Solid Edge part; units mm, degrees
sketch "Sketch1" plane through (0, 0, 0) normal (0, -1, 0) x (1, 0, 0)
  line L0 (20, 36) -> (-16, 36)
  line L1 (-16, 36) -> (-16, -36)
  line L2 (-16, -36) -> (20, -36)
  line L3 (20, -36) -> (20, -40)
  line L4 (20, -40) -> (-20, -40)
  line L5 (-20, -40) -> (-20, 40)
  line L6 (-20, 40) -> (20, 40)
  line L7 (20, 40) -> (20, 36)
  dimension "D1" = 20
  dimension "D2" = 20
  dimension "D3" = 20
extrude "Protrusion1" add sketch "Sketch1" against normal blind 350
sketch "Sketch2" plane through (0, 175, 40) normal (0, 0, 1) x (0, 1, 0)
  line L0 (-175, 20) -> (-135, -20)
extrude "Cutout1" cut sketch "Sketch2" against normal through all material side at (0.0354, 19.9646, 40)
sketch "Sketch3" plane through (0, 175, 40) normal (0, 0, 1) x (0, 1, 0)
  line L0 (175, 20) -> (135, -20)
extrude "Cutout2" cut sketch "Sketch3" against normal through all material side at (0.0354, 330.0354, 40)
hole "Bohrung_1" at (-16, 142.5, 17) direction (-1, 0, 0) diameter 6 end up to next
hole "Hole1" at (-16, 207.5, 17) direction (-1, 0, 0) diameter 6 end up to next
hole "Bohrung_3" at (-16, 50, 15.6) direction (-1, 0, 0) diameter 5 end up to next
hole "Hole2" at (-16, 105, 15.6) direction (-1, 0, 0) diameter 5 end up to next
hole "Hole3" at (-16, 245, 15.6) direction (-1, 0, 0) diameter 5 end up to next
hole "Hole4" at (-16, 300, 15.6) direction (-1, 0, 0) diameter 5 end up to next
sketch "Sketch4" plane through (20, 175, -38) normal (1, 0, 0) x (0, 1, 0)
  line L0 (-25, -2) -> (25, -2)
  line L1 (25, -2) -> (25, 28)
  line L2 (25, 28) -> (-25, 28)
  line L3 (-25, 28) -> (-25, -2)
  dimension "D1" = 25
  dimension "D2" = 25
extrude "Cutout3" cut sketch "Sketch4" against normal through all
properties material "AlMgSi 0,5-1"
Geometry: final body of the model. Coordinates: model frame, mm. A direction names the side the tool comes from. Coordinates: 2 decimals unless noted, no trailing zeros. Order: outer loops, then holes, each group sorted by start corner. A loop starts at its lowest first (then second) coordinate and runs counter-clockwise, first axis right, second up.
(1) Material intervals for probe 1 along Z at (x, y) = (-18.6, 245); probe 2 along Z at (x, y) = (-16.9, 207.5); probe 3 along X at (y, z) = (230, 33), sorted ascending.
(2) Section query A-A (z = -23). Return the cut outline in (x, y).
(3) Section query C-C (x = -8). Return the cut outline in (y, z), plus the area to 3 significant figures.
(4) First-contact query: pin 1 (6 mm diameter, centred on y = 105, z = 15.6, fed in from +X); pin 2 (9 mm diameter, centred on x = -2, z = -32.5, fed in from +Y); pin 3 (2 mm diameter, centred on x = -17.5, y = 163.5, fed in from -Z). Flat tips, straight axial feed; report the tip coordinate or a pass-through.
(5) Draft query along Y for faces 4 (the face through (-16.4, 346.4, 0.2)), 5 (the face through (-20, 173, -1)), 6 (the face through (-17.972, 210.474, 17.391)). Return one class per face: pulls with the +Y half, pulls with the -Y half, needs draft (parallel to the pull), parting line crosses it, or undercut.
(6) Access query for faces 1 (the face through (2, 173, 36)), 2 (the face through (-17.97, 145.03, 15.39)), 3 (the face through (-5.8, 200, -36.2)). Directions: +Z, -Z, +X, -X, +Y, -Y. A direction counts if a zero-diameter tool reaches every point of the face in a straight line with its end or side. Return the directions, or none.
(7) Section query B-B (y = 142.5). Return the cut outline in (x, z), plus the area to 3 significant figures.
(8) Section query D-D (y = 84). Return the cut outline in (x, z).
Solution:
1. probe 1: z = -40 to 13.1, 18.1 to 40
1. probe 2: z = -40 to 14, 20 to 40
1. probe 3: x = -20 to -16
2. outline: (-20, 0) - (-16, 4) - (-16, 150) - (-20, 150) - close; (-20, 200) - (-16, 200) - (-16, 346) - (-20, 350) - close
3. outline: (12, -40) - (150, -40) - (150, -36) - (12, -36) - close; (12, 36) - (338, 36) - (338, 40) - (12, 40) - close; (200, -40) - (338, -40) - (338, -36) - (200, -36) - close
3. area: 2,410 mm2
4. pin 1: stops at x = -16
4. pin 2: stops at y = 334.83
4. pin 3: stops at z = -10
5. face 4: pulls with the +Y half
5. face 5: needs draft
5. face 6: undercut
6. face 1: +X, +Y, -Y
6. face 2: +X, -X
6. face 3: -Z, +X, -X
7. outline: (-20, -40) - (20, -40) - (20, -36) - (-16, -36) - (-16, 14) - (-20, 14) - close; (-20, 20) - (-16, 20) - (-16, 36) - (20, 36) - (20, 40) - (-20, 40) - close
7. area: 584 mm2
8. outline: (-20, -40) - (20, -40) - (20, -36) - (-16, -36) - (-16, 36) - (20, 36) - (20, 40) - (-20, 40) - close
